Source: three-view drawing plus pictorial views. Frame: mm from the lowest corner of the part. A direction names the side the tool comes from. Round coordinates to 2 decimals unless told otherwise and drop trailing zeros. Loops run counter-clockwise (first coordinate to the right, second up) from the corner with the lowest first, then second, coordinate; pieces in that order, holes last. Notation, with made-up numbers: M 55,38 L 70,38 A31 ccw 70,77 Z; hole C 25,-35 d6. An arc over 180 degrees is marked long. Return JSON: item names as keys, results as strings. Group by question number.
1) Contact query for flat-ended pins moving along their axis: P1, Ø1, axis at x = 5, z = 1.5, coming from the -Y side; P2, Ø4, axis at x = 2.5, y = 2.5, coming from the -Z side. Output: stop coordinate, or through.
2) Mould query, pull axis X, two halves, no side actions, for the marked faces 3, 4, 5 and 6. Classes: +X half, -X half, draft (parallel to the pull), parting line (faces both ways), or undercut.
3) Section C-C (z = 3.65). Output: boundary loops of the cut face in (x, y), plus the area to 3 significant figures.
4) Access query for the marked faces 1 and 2. Directions: +Z, -Z, +X, -X, +Y, -Y. A direction counts if a zero-diameter tool reaches every point of the face in a straight line with its end or side. Return the directions, or none.
5) Section B-B (x = 3.55). Output: boundary loops of the cut face in (y, z).
6) Material intervals for line 1 (Y direction, x = 3.55, z = 1.85); line 2 (Y direction, x = 2.75, z = 2.1) (1 decimal); line 3 (Z direction, x = 2, y = 5.25), sorted ascending. Write a range as from..to.
7) Section A-A (z = 2.15). Output: boundary loops of the cut face in (x, y).
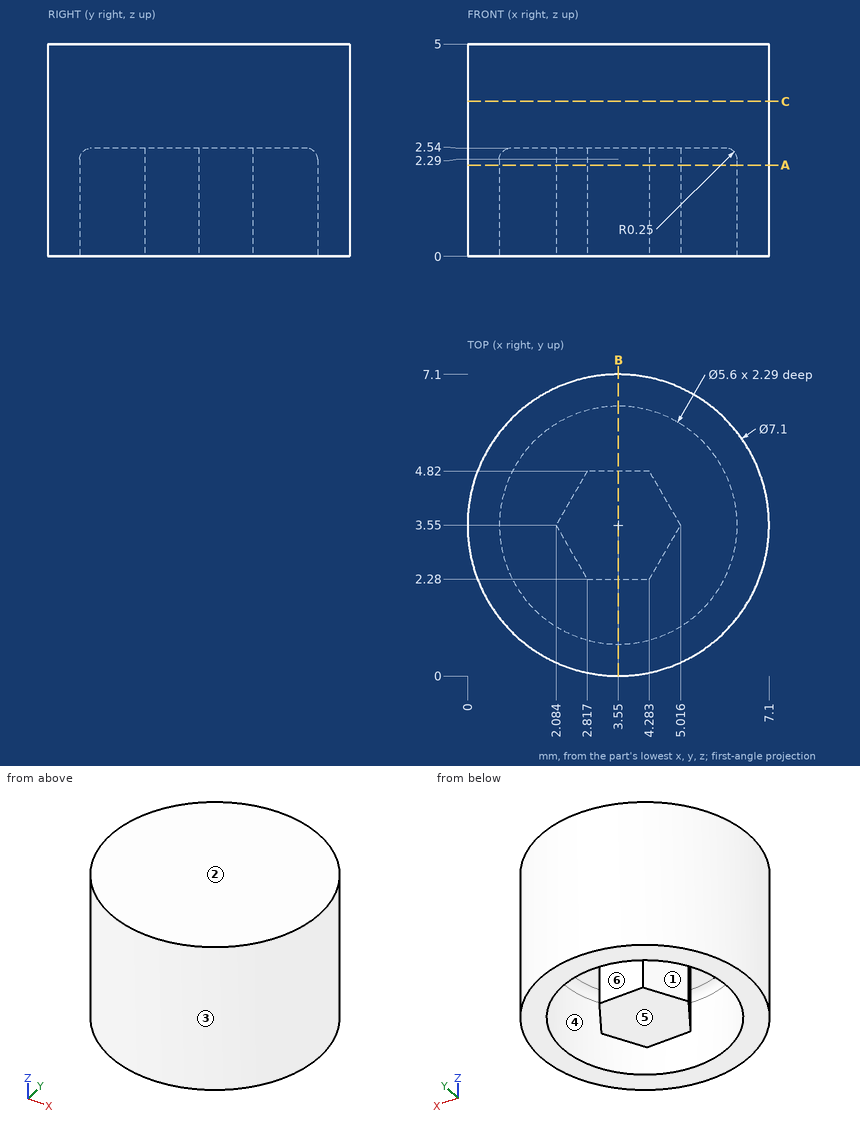
Returned:
{
 "1": {"P1": "stops at y = 0.13", "P2": "stops at z = 0"},
 "2": {"face 3": "parting line", "face 4": "undercut", "face 5": "draft", "face 6": "undercut"},
 "3": {"outline": "C 3.55,3.55 d7.1", "area": "39.6 mm^2"},
 "4": {"face 1": "-Z", "face 2": "+Z, +X, -X, +Y, -Y"},
 "5": {"outline": "M 0,0 L 0.75,0 L 0.75,2.29 A0.25 cw 1,2.54 L 2.28,2.54 L 2.28,0 L 4.82,0 L 4.82,2.54 L 6.1,2.54 A0.25 cw 6.35,2.29 L 6.35,0 L 7.1,0 L 7.1,5 L 0,5 Z"},
 "6": {"line 1": "y = 0..0.75, 2.28..4.82, 6.35..7.1", "line 2": "y = 0.1..0.9, 2.4..4.7, 6.2..7", "line 3": "z = 2.54..5"},
 "7": {"outline": "C 3.55,3.55 d7.1; M 2.08,3.55 L 2.82,2.28 L 4.28,2.28 L 5.02,3.55 L 4.28,4.82 L 2.82,4.82 Z; hole C 3.55,3.55 d5.6"}
}
